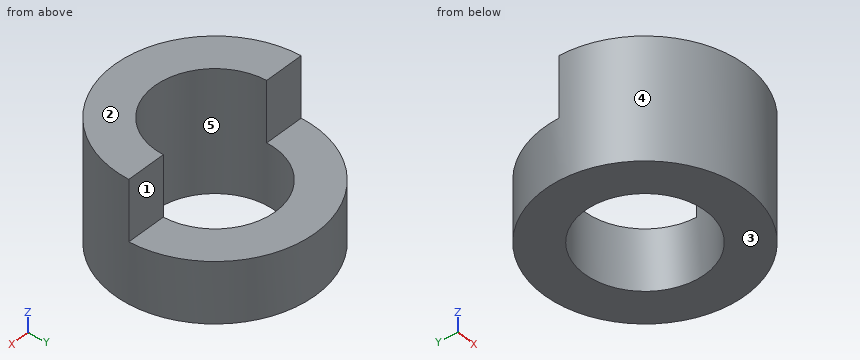
from build123d import *

# Parameters (mm, degrees)
SKETCH1_R           = 50
BOSS_EXTRUDE1_DEPTH = 60
SKETCH2_R           = 30
CUT_EXTRUDE1_DEPTH  = 60
CUT_EXTRUDE2_DEPTH  = 30


with BuildPart() as part:
    # Sketch1 → Boss-Extrude1 (new body)
    with BuildSketch(Plane.XY):
        Circle(SKETCH1_R)
    extrude(amount=BOSS_EXTRUDE1_DEPTH)

    # Sketch2 → Cut-Extrude1 (cut)
    with BuildSketch(Plane.XY.offset(60)):
        Circle(SKETCH2_R)
    extrude(amount=-CUT_EXTRUDE1_DEPTH, mode=Mode.SUBTRACT)

    # Sketch3 → Cut-Extrude2 (cut)
    with BuildSketch(Plane.XY.offset(60)):
        with BuildLine():
            Line((-50, 0), (-30, 0))
            ThreePointArc((-30, 0), (0, 30), (30, 0))
            Line((30, 0), (50, 0))
            ThreePointArc((50, 0), (0, 50), (-50, 0))
        make_face()
    extrude(amount=-CUT_EXTRUDE2_DEPTH, mode=Mode.SUBTRACT)


solid = part.part
Verification items for the finished model (mm, model axes). Face numbers are marked on the shaded views. A direction names the side the tool comes from. Coordinates: 2 decimals unless noted, no trailing zeros. Order: outer loops, then holes, each group sorted by start corner. A loop starts at its lowest first (then second) coordinate and runs counter-clockwise, first axis right, second up. Notation, with made-up numbers: M -23,-25 L -14,-25 A6 ccw -14,-19 Z; hole C 11,50 d3. An arc over 180 degrees is marked long. Return JSON: item names as keys, results as strings.
1) Cross-section at A-A, the plane x = 0. Record the boundary of the cut face in (y, z), and give its area (3 significant figures).
Answer list:
{"outline": "M -50,0 L -30,0 L -30,60 L -50,60 Z; M 30,0 L 50,0 L 50,30 L 30,30 Z", "area": "1,800 mm2"}
2) Access from +Z, -Z, +X, -X, +Y, -Y to the whole of each face (thin tool, end or side, straight path). Record for the marked faces 1 and 2.
Answer list:
{"face 1": "+Z, +X, -X, +Y", "face 2": "+Z, +X, -X, +Y, -Y"}
3) Cross-section at C-C, the plane z = 20.5. Record the boundary of the cut face in (x, y).
Answer list:
{"outline": "C 0,0 d100; hole C 0,0 d60"}
4) Cross-section at D-D, the plane z = 52.5. Record the boundary of the cut face in (x, y).
Answer list:
{"outline": "M -50,0 A50 ccw 50,0 L 30,0 A30 cw -30,0 Z"}
5) Cross-section at B-B, the plane y = 21. Record the boundary of the cut face in (x, z).
Answer list:
{"outline": "M -45.38,0 L -21.42,0 L -21.42,30 L -45.38,30 Z; M 21.42,0 L 45.38,0 L 45.38,30 L 21.42,30 Z"}
6) Gauge pin test, flat ends, axial feed: pin 1 (16 mm diameter, centred on x = -37, z = 40.5, fed in from +Y); pin 2 (8 mm diameter, centred on x = -5, z = 35.5, fed in from +Y); pin 3 (6 mm diameter, centred on x = 13, z = 20, fed in from +Y). Record the tip position at first contact, or that the pin passes through.
Answer list:
{"pin 1": "y = 0", "pin 2": "y = -28.62", "pin 3": "y = 48.99"}
7) Release check for a two-part mould opening along Y. For the marked faces 3, 4 and 5 record: +Y half, -Y half, draft (parallel to the pull), parting line (faces both ways), or undercut.
Answer list:
{"face 3": "draft", "face 4": "parting line", "face 5": "undercut"}
8) Thickness scan on L1, parallel to Y at x = 0, z = 19; L2, parallel to Z at x = -41, y = 17; L3, parallel to Y at x = -2, z = 3. Record the ranges inside material, lowest first. Write a range as [from, to].
Answer list:
{"L1": "[-50, -30], [30, 50]", "L2": "[0, 30]", "L3": "[-49.96, -29.93], [29.93, 49.96]"}
